Here's how the part is built. I have some questions about the finished solid (model axes, mm). Give positions to 0.01 mm unless a question says otherwise; leave off trailing zeros. Order: outer loops, then holes, each group sorted by start corner. A loop starts at its lowest first (then second) coordinate and runs counter-clockwise, first axis right, second up. Notation, with made-up numbers: M 38.25,44.5 L 46.25,44.5 A13 cw 46.25,63.5 Z; hole C 34,47 d5. An arc over 180 degrees is marked long. Use one line per item in the form item = value.
Autodesk Inventor part; units mm, degrees
ref_plane "YZ Plane" through (0, 0, 0) normal (1, 0, 0) x (0, 1, 0)
ref_plane "XZ Plane" through (0, 0, 0) normal (0, 1, 0) x (-1, 0, 0)
ref_plane "XY Plane" through (0, 0, 0) normal (0, 0, 1) x (1, 0, 0)
sketch "Sketch1" plane through (0, 0, 0) normal (0, 1, 0) x (-1, 0, 0)
  line L0 (80, 52) -> (-80, 52)
  line L1 (-80, 52) -> (-80, -52)
  line L2 (-80, -52) -> (80, -52)
  line L3 (80, -52) -> (80, 52)
  line L4 (80, 52) -> (-80, -52) construction
  line L5 (-80, 52) -> (80, -52) construction
  point P0 (0, 0)
  dimension "d0" = 160
  dimension "d1" = 104
extrude "Extrusion1" add sketch "Sketch1" along normal blind 12
sketch "Sketch2" plane through (0, 12, 0) normal (0, 1, 0) x (1, 0, 0)
  line L0 (-80, 52) -> (-80, -52)
  line L1 (80, 52) -> (-80, 52)
  line L2 (-38.25, 26.5) -> (-38.25, 11)
  line L3 (-60.75, 11) -> (-60.75, 26.5)
  arc A0 (-38.25, 26.5) -> (-60.75, 26.5) centre (-49.5, 18.75) ccw
  arc A1 (-60.75, 11) -> (-38.25, 11) centre (-49.5, 18.75) ccw
  point P0 (0, 0)
  dimension "d33" = 22.5
  dimension "d34" = 15.5
  dimension "d35" = 19.25
  dimension "d37" = 33.25
  dimension "d38" = 7.75
extrude "Extrusion2" cut sketch "Sketch2" against normal up to next
pattern_linear "Rectangular Pattern1" count 4 spacing -32.5 along (-1, 0, 0) count 2 spacing 37.5 along (0, 0, 1) of "Extrusion2"
sketch "Sketch4" plane through (0, 12, 0) normal (0, 1, 0) x (1, 0, 0)
  line L0 (-80, 52) -> (-80, -52)
  line L1 (80, 52) -> (-80, 52)
  line L2 (80, -52) -> (80, 52)
  line L3 (-80, -52) -> (80, -52)
  point P0 (0, 0)
  point P1 (-67.5, 39.5)
  point P2 (67.5, 39.5)
  point P3 (67.5, -39.5)
  point P4 (-67.5, -39.5)
  dimension "d24" = 12.5
  dimension "d25" = 12.5
  dimension "d26" = 12.5
  dimension "d27" = 12.5
  dimension "d28" = 12.5
  dimension "d29" = 12.5
  dimension "d30" = 12.5
  dimension "d31" = 12.5
hole "Hole1" at (-67.5, 12, -39.5) at (67.5, 12, -39.5) at (67.5, 12, 39.5) at (-67.5, 12, 39.5) direction (0, -1, 0) diameter 6.756 depth 25.4
fillet "Fillet1" radius 2 4 edges at (-80, 6, 52) (80, 6, 52) (80, 6, -52) (-80, 6, -52)
properties part number "4_OM_VialPlate_0.5mmReduce"
Q1. I'm going to push a flat-ended pin straight in: pin 1 Ø6 at (x, z) = (67.5, -39.5) entering from -Y. Where does the tip first touch, or does it pass through?
Found:
pin_1 = through
Q2. I want a section at A-A on z = 17. Write out the boundary of the cut face in (x, y), then the cut area to 3 significant figures.
Found:
outline = M -80,0 L -60.75,0 L -60.75,12 L -80,12 Z; M -38.25,0 L -28.25,0 L -28.25,12 L -38.25,12 Z; M -5.75,0 L 4.25,0 L 4.25,12 L -5.75,12 Z; M 26.75,0 L 36.75,0 L 36.75,12 L 26.75,12 Z; M 59.25,0 L 80,0 L 80,12 L 59.25,12 Z
area = 840 mm²
Q3. I need wall thicknesses on L1, parallel to Z at x = 67.5, y = 5.75; L2, parallel to X at y = 5.25, z = 24; L3, parallel to X at y = 3, z = 39.5. Which ranges of each line are inside material? Lowest first, please.
Found:
L1 = -52 to -42.88, -36.12 to 36.12, 42.88 to 52
L2 = -80 to -60.75, -38.25 to -28.25, -5.75 to 4.25, 26.75 to 36.75, 59.25 to 80
L3 = -80 to -70.88, -64.12 to 64.12, 70.88 to 80
Q4. I want a section at C-C on x = -56. Write out the boundary of the cut face in (y, z).
Found:
outline = M 0,-52 L 12,-52 L 12,-30.77 L 0,-30.77 Z; M 0,-6.73 L 12,-6.73 L 12,6.73 L 0,6.73 Z; M 0,30.77 L 12,30.77 L 12,52 L 0,52 Z
Q5. I want a section at B-B on z = -39.5. Write out the boundary of the cut face in (x, y).
Found:
outline = M -80,0 L -70.88,0 L -70.88,12 L -80,12 Z; M -64.12,0 L 64.12,0 L 64.12,12 L -64.12,12 Z; M 70.88,0 L 80,0 L 80,12 L 70.88,12 Z
Q6. I want a section at D-D on y = 8.75. State how many separate pieces and enclosed holes the cut face has, then the cut area to 3 significant figures.
Found:
separate_pieces = 1
enclosed_holes = 12
area = 12,200 mm²
